The listing builds one solid part. Answer for the finished solid, in the listing's coordinates (mm). Face numbers are marked on the shaded views. A direction names the side the tool comes from. Give positions to 0.01 mm unless a question says otherwise; leave off trailing zeros. Order: outer loops, then holes, each group sorted by start corner. A loop starts at its lowest first (then second) coordinate and runs counter-clockwise, first axis right, second up. Notation, with made-up numbers: (-32.5, 50) - (-23.5, 50) arc R19 cw to (-23.5, 71) - close; hole circle Ø7 at (75.25, 73). An arc over 180 degrees is marked (long way). Use CSV: the item, a comma, the result in double quotes.
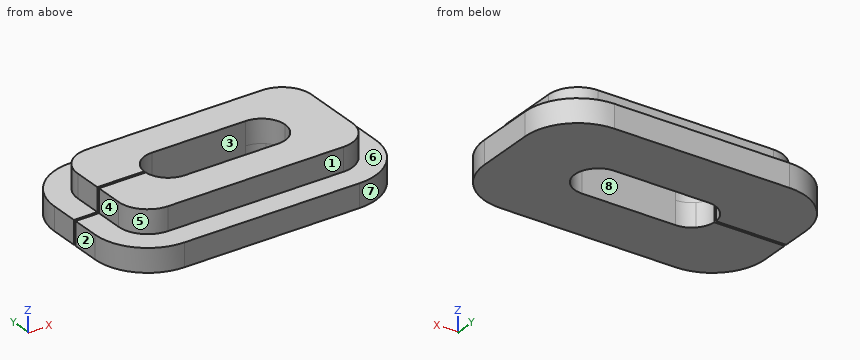
```python
from build123d import *
from build123d.topology import SkipClean

# Parameters (mm, degrees)
SKETCH1_W               = 20
SKETCH1_H               = 10
SKETCH1_W_2             = 12
SKETCH1_H_2             = 4
BOSS_EXTRUDE1_DEPTH     = 2
FILLET1_R               = 2.5
BOSS_EXTRUDE2_DEPTH     = 2
CUT_EXTRUDE1_DEPTH      = 15.035668848
CUT_EXTRUDE1_DEPTH_BACK = 15.035668848
SKETCH3_W               = 8
SKETCH3_H               = 0.2


with BuildPart() as part:
    # Sketch1 → Boss-Extrude1 (new body)
    # profile 1 of 5: a face of its own
    with BuildSketch(Plane.XY):
        Rectangle(SKETCH1_W, SKETCH1_H)
        Rectangle(SKETCH1_W_2, SKETCH1_H_2, mode=Mode.SUBTRACT)
    # profile 2 of 5: a face of its own
    with BuildSketch(Plane.XY):
        with BuildLine():
            ThreePointArc((-6, 0), (-5.414213562, 1.414213562), (-4, 2))
            Line((-4, 2), (-6, 2))
            Line((-6, 2), (-6, 0))
        make_face()
    # profile 3 of 5: a face of its own
    with BuildSketch(Plane.XY):
        with BuildLine():
            ThreePointArc((-4, -2), (-5.414213562, -1.414213562), (-6, 0))
            Line((-6, 0), (-6, -2))
            Line((-6, -2), (-4, -2))
        make_face()
    # profile 4 of 5: a face of its own
    with BuildSketch(Plane.XY):
        with BuildLine():
            Line((6, -2), (6, 0))
            ThreePointArc((6, 0), (5.414213562, -1.414213562), (4, -2))
            Line((4, -2), (6, -2))
        make_face()
    # profile 5 of 5: a face of its own
    with BuildSketch(Plane.XY):
        with BuildLine():
            Line((6, 0), (6, 2))
            Line((6, 2), (4, 2))
            ThreePointArc((4, 2), (5.414213562, 1.414213562), (6, 0))
        make_face()
    extrude(amount=BOSS_EXTRUDE1_DEPTH)

    # Fillet1
    fillet1_edges = [part.edges().sort_by_distance(p)[0] for p in [
        (10, -5, 1),
        (-10, -5, 1),
        (-10, 5, 1),
        (10, 5, 1),
    ]]
    fillet(fillet1_edges, radius=FILLET1_R)

    # Sketch2 → Boss-Extrude2 (add)
    with SkipClean():  # the faces are left unmerged after this step: merging them gives an invalid solid
        with BuildSketch(Plane(origin=(0, 0, 0), x_dir=(-1, 0, 0), z_dir=(0, 0, -1))):
            with BuildLine():
                Line((-3.758342613, 5), (3.758342613, 5))
                ThreePointArc((3.758342613, 5), (5.378679665, 6.468626971), (7.500000019, 7))
                Line((7.500000019, 7), (-7.5, 7))
                ThreePointArc((-7.5, 7), (-5.378679656, 6.468626967), (-3.758342613, 5))
            make_face()
            with BuildLine():
                ThreePointArc((-11.241657387, 0), (-10.681980515, 0.681980515), (-10, 1.241657387))
                Line((-10, 1.241657387), (-10, 2.5))
                ThreePointArc((-10, 2.5), (-9.267766953, 4.267766953), (-7.5, 5))
                Line((-7.5, 5), (-3.758342613, 5))
                ThreePointArc((-3.758342613, 5), (-5.378679656, 6.468626967), (-7.5, 7))
                ThreePointArc((-7.5, 7), (-10.681980515, 5.681980515), (-12, 2.5))
                ThreePointArc((-12, 2.5), (-11.80624304, 1.19375696), (-11.241657387, 0))
            make_face()
            with BuildLine():
                Line((-10, -1.241657387), (-10, 1.241657387))
                ThreePointArc((-10, 1.241657387), (-10.681980515, 0.681980515), (-11.241657387, 0))
                ThreePointArc((-11.241657387, 0), (-10.681980515, -0.681980515), (-10, -1.241657387))
            make_face()
            with BuildLine():
                ThreePointArc((-12, -2.5), (-11.80624304, -1.19375696), (-11.241657387, 0))
                ThreePointArc((-11.241657387, 0), (-11.80624304, 1.19375696), (-12, 2.5))
                Line((-12, 2.5), (-12, -2.5))
            make_face()
            with BuildLine():
                Line((-10, -2.5), (-10, -1.241657387))
                ThreePointArc((-10, -1.241657387), (-10.681980515, -0.681980515), (-11.241657387, 0))
                ThreePointArc((-11.241657387, 0), (-11.80624304, -1.19375696), (-12, -2.5))
                ThreePointArc((-12, -2.5), (-10.681980515, -5.681980515), (-7.5, -7))
                ThreePointArc((-7.5, -7), (-5.378679656, -6.468626967), (-3.758342613, -5))
                Line((-3.758342613, -5), (-7.5, -5))
                ThreePointArc((-7.5, -5), (-9.267766953, -4.267766953), (-10, -2.5))
            make_face()
            with BuildLine():
                ThreePointArc((7.499999979, -7), (5.378679647, -6.468626962), (3.758342613, -5))
                Line((3.758342613, -5), (-3.758342613, -5))
                ThreePointArc((-3.758342613, -5), (-5.378679656, -6.468626967), (-7.5, -7))
                Line((-7.5, -7), (7.499999979, -7))
            make_face()
            with BuildLine():
                Line((7.5, -5), (3.758342613, -5))
                ThreePointArc((3.758342613, -5), (5.378679647, -6.468626962), (7.499999979, -7))
                ThreePointArc((7.499999979, -7), (10.681980508, -5.681980523), (12, -2.5))
                ThreePointArc((12, -2.5), (11.80624304, -1.19375696), (11.241657387, 0))
                ThreePointArc((11.241657387, 0), (10.681980515, -0.681980515), (10, -1.241657387))
                Line((10, -1.241657387), (10, -2.5))
                ThreePointArc((10, -2.5), (9.267766953, -4.267766953), (7.5, -5))
            make_face()
            with BuildLine():
                ThreePointArc((11.241657387, 0), (10.681980515, 0.681980515), (10, 1.241657387))
                Line((10, 1.241657387), (10, -1.241657387))
                ThreePointArc((10, -1.241657387), (10.681980515, -0.681980515), (11.241657387, 0))
            make_face()
            with BuildLine():
                Line((12, -2.5), (12, 2.5))
                ThreePointArc((12, 2.5), (11.80624304, 1.19375696), (11.241657387, 0))
                ThreePointArc((11.241657387, 0), (11.80624304, -1.19375696), (12, -2.5))
            make_face()
            with BuildLine():
                ThreePointArc((7.500000019, 7), (5.378679665, 6.468626971), (3.758342613, 5))
                Line((3.758342613, 5), (7.5, 5))
                ThreePointArc((7.5, 5), (9.267766953, 4.267766953), (10, 2.5))
                Line((10, 2.5), (10, 1.241657387))
                ThreePointArc((10, 1.241657387), (10.681980515, 0.681980515), (11.241657387, 0))
                ThreePointArc((11.241657387, 0), (11.80624304, 1.19375696), (12, 2.5))
                ThreePointArc((12, 2.5), (10.681980522, 5.681980509), (7.500000019, 7))
            make_face()
            with BuildLine():
                ThreePointArc((-5.365330412, 1.461462577), (-4.73385109, 1.860500625), (-4, 2))
                Line((-4, 2), (-3.027864045, 2))
                ThreePointArc((-3.027864045, 2), (-3.006971411, 2.249612098), (-3, 2.5))
                ThreePointArc((-3, 2.5), (-3.19375696, 3.80624304), (-3.758342613, 5))
                Line((-3.758342613, 5), (-7.5, 5))
                ThreePointArc((-7.5, 5), (-9.267766953, 4.267766953), (-10, 2.5))
                Line((-10, 2.5), (-10, 1.241657387))
                ThreePointArc((-10, 1.241657387), (-7.7131787, 1.994947702), (-5.365330412, 1.461462577))
            make_face()
            with BuildLine():
                ThreePointArc((-5.365330412, -1.461462577), (-6, 0), (-5.365330412, 1.461462577))
                ThreePointArc((-5.365330412, 1.461462577), (-7.7131787, 1.994947702), (-10, 1.241657387))
                Line((-10, 1.241657387), (-10, -1.241657387))
                ThreePointArc((-10, -1.241657387), (-7.7131787, -1.994947702), (-5.365330412, -1.461462577))
            make_face()
            with BuildLine():
                ThreePointArc((-4, -2), (-4.73385109, -1.860500625), (-5.365330412, -1.461462577))
                ThreePointArc((-5.365330412, -1.461462577), (-7.7131787, -1.994947702), (-10, -1.241657387))
                Line((-10, -1.241657387), (-10, -2.5))
                ThreePointArc((-10, -2.5), (-9.267766953, -4.267766953), (-7.5, -5))
                Line((-7.5, -5), (-3.758342613, -5))
                ThreePointArc((-3.758342613, -5), (-3.19375696, -3.80624304), (-3, -2.5))
                ThreePointArc((-3, -2.5), (-3.006971411, -2.249612098), (-3.027864045, -2))
                Line((-3.027864045, -2), (-4, -2))
            make_face()
            with BuildLine():
                Line((3.027864045, -2), (-3.027864045, -2))
                ThreePointArc((-3.027864045, -2), (-3.006971411, -2.249612098), (-3, -2.5))
                ThreePointArc((-3, -2.5), (-3.19375696, -3.80624304), (-3.758342613, -5))
                Line((-3.758342613, -5), (3.758342613, -5))
                ThreePointArc((3.758342613, -5), (3.127746546, -3.564612481), (3.027864045, -2))
            make_face()
            with BuildLine():
                Line((4, -2), (3.027864045, -2))
                ThreePointArc((3.027864045, -2), (3.127746546, -3.564612481), (3.758342613, -5))
                Line((3.758342613, -5), (7.5, -5))
                ThreePointArc((7.5, -5), (9.267766953, -4.267766953), (10, -2.5))
                Line((10, -2.5), (10, -1.241657387))
                ThreePointArc((10, -1.241657387), (7.7131787, -1.994947702), (5.365330412, -1.461462577))
                ThreePointArc((5.365330412, -1.461462577), (4.73385109, -1.860500625), (4, -2))
            make_face()
            with BuildLine():
                ThreePointArc((10, 1.241657387), (7.7131787, 1.994947702), (5.365330412, 1.461462577))
                ThreePointArc((5.365330412, 1.461462577), (6, 0), (5.365330412, -1.461462577))
                ThreePointArc((5.365330412, -1.461462577), (7.7131787, -1.994947702), (10, -1.241657387))
                Line((10, -1.241657387), (10, 1.241657387))
            make_face()
            with BuildLine():
                ThreePointArc((3.758342613, 5), (3.127746546, 3.564612481), (3.027864045, 2))
                Line((3.027864045, 2), (4, 2))
                ThreePointArc((4, 2), (4.73385109, 1.860500625), (5.365330412, 1.461462577))
                ThreePointArc((5.365330412, 1.461462577), (7.7131787, 1.994947702), (10, 1.241657387))
                Line((10, 1.241657387), (10, 2.5))
                ThreePointArc((10, 2.5), (9.267766953, 4.267766953), (7.5, 5))
                Line((7.5, 5), (3.758342613, 5))
            make_face()
            with BuildLine():
                ThreePointArc((-3, 2.5), (-3.006971411, 2.249612098), (-3.027864045, 2))
                Line((-3.027864045, 2), (3.027864045, 2))
                ThreePointArc((3.027864045, 2), (3.127746546, 3.564612481), (3.758342613, 5))
                Line((3.758342613, 5), (-3.758342613, 5))
                ThreePointArc((-3.758342613, 5), (-3.19375696, 3.80624304), (-3, 2.5))
            make_face()
        extrude(amount=BOSS_EXTRUDE2_DEPTH)

    # Sketch3 → Cut-Extrude1 (cut, two sides: drawn at the far end of the back side and taken through both)
    with SkipClean():  # the faces are left unmerged after this step: merging them gives an invalid solid
        with BuildSketch(Plane.XY.offset(-CUT_EXTRUDE1_DEPTH_BACK)):
            with Locations((-8, 0)):
                Rectangle(SKETCH3_W, SKETCH3_H)
        extrude(amount=CUT_EXTRUDE1_DEPTH + CUT_EXTRUDE1_DEPTH_BACK, mode=Mode.SUBTRACT)


solid = part.part
```
Item 1: Find the intervals of material crossed by line 1 along Y through (x, z) = (-3, -1.35); line 2 along Y through (x, z) = (-7.5, 0.65); line 3 along Z through (x, y) = (10.25, -6), in increasing order.
Taken from the geometry:
line 1,"-7 to -2, 2 to 7"
line 2,"-5 to -0.1, 0.1 to 5"
line 3,"-2 to 0"
Item 2: Each of these flat-tipped pins is pushed along its axis until it touches: pin 1 (1.5 mm diameter, centred on y = -4.5, z = 1, fed in from +X); pin 2 (0.6 mm diameter, centred on x = 1, z = 1.5, fed in from -Y); pin 3 (1.6 mm diameter, centred on y = -1, z = 1, fed in from +X). Where does it stop, or does it pass through?
Taken from the geometry:
pin 1,"x = 9.67"
pin 2,"y = -5"
pin 3,"x = 10"
Item 3: Which of the six approach directions +Z, -Z, +X, -X, +Y, -Y give full straight-line access (tool end or side, diameter ignored) to the marked faces 1, 2, 3, 4 and 5?
Taken from the geometry:
face 1,"+Z, +X, -X, -Y"
face 2,"+Z, -Z, -X, +Y, -Y"
face 3,"+Z, -Z"
face 4,"+Z, -X, +Y, -Y"
face 5,"+Z, -X, -Y"
Item 4: The part is cut by section B-B (z = -1.55). Give the vertices of the cut face in (x, y).
Taken from the geometry:
outline,"(-12, -2.5) arc R4.5 ccw to (-7.5, -7) - (7.5, -7) arc R4.5 ccw to (12, -2.5) - (12, 2.5) arc R4.5 ccw to (7.5, 7) - (-7.5, 7) arc R4.5 ccw to (-12, 2.5) - (-12, 0.1) - (-6, 0.1) arc R2 cw to (-4, 2) - (4, 2) arc R2 cw to (4, -2) - (-4, -2) arc R2 cw to (-6, -0.1) - (-12, -0.1) - close"
Item 5: The part is cut by section A-A (x = -8.5). Give the vertices of the cut face in (y, z), and give its area (3 significant figures).
Taken from the geometry:
outline,"(-6.89, -2) - (-0.1, -2) - (-0.1, 2) - (-4.79, 2) - (-4.79, 0) - (-6.89, 0) - close; (0.1, -2) - (6.89, -2) - (6.89, 0) - (4.79, 0) - (4.79, 2) - (0.1, 2) - close"
area,"45.9 mm^2"
Item 6: The mould has two halves that part along Y. Classify the marked faces 6, 7 and 8: +Y half, -Y half, draft (parallel to the pull), parting line (faces both ways), or undercut.
Taken from the geometry:
face 6,"draft"
face 7,"-Y half"
face 8,"undercut"
Item 7: The part is cut by section C-C (y = -1.75). Give the vertices of the cut face in (x, z).
Taken from the geometry:
outline,"(-12, -2) - (-4.97, -2) - (-4.97, 2) - (-10, 2) - (-10, 0) - (-12, 0) - close; (4.97, -2) - (12, -2) - (12, 0) - (10, 0) - (10, 2) - (4.97, 2) - close"
Item 8: The part is cut by section D-D (x = 6.25). Give the vertices of the cut face in (y, z), and give its area (3 significant figures).
Taken from the geometry:
outline,"(-7, -2) - (7, -2) - (7, 0) - (5, 0) - (5, 2) - (-5, 2) - (-5, 0) - (-7, 0) - close"
area,"48.0 mm^2"
